Source: CAD feature listing. Evaluate the final solid. Frame: model axes, mm. A direction names the side the tool comes from. Give positions to 0.01 mm unless a question says otherwise; leave off trailing zeros. Loops run counter-clockwise (first coordinate to the right, second up) from the corner with the lowest first, then second, coordinate; pieces in that order, holes last. Notation, with made-up numbers: (40, -21) -> (83, -21) arc R9 cw to (83, -4) -> close; hole circle Ø10 at (44, -22). An arc over 180 degrees is marked (long way). Return JSON: item names as keys, results as strings. Group by question number.
```python
from build123d import *

# Parameters (mm, degrees)
SKETCH_1_W          = 25
SKETCH_1_H          = 10
EXTRUDE_1_DEPTH     = 3
EXTRUDE_3_DEPTH     = 7
EXTRUDE_4_DEPTH     = 39
EXTRUDE_6_DEPTH     = 3
EXTRUDE_7_DEPTH     = 3
SKETCH_10_W         = 25
SKETCH_10_H         = 10
CUT_EXTRUDE_1_DEPTH = 3
FILLET_1_R          = 5
FILLET_2_R          = 5
SKETCH_12_W         = 9
SKETCH_12_H         = 1.5
EXTRUDE_9_DEPTH     = 4
FILLET_3_R          = 5


with BuildPart() as part:
    # 草图1 → 凸台-拉伸1 (new body)
    with BuildSketch(Plane.XY):
        with Locations((12.5, -5)):
            Rectangle(SKETCH_1_W, SKETCH_1_H)
    extrude(amount=EXTRUDE_1_DEPTH)

    # 草图5 → 凸台-拉伸3 (add)
    with BuildSketch(Plane.XY.offset(3)):
        Polygon((25, 0), (-2, 0), (-8, 0), (-8, -3), (0, -3), (27.572478777, -3), (31, -3), (31, 0), align=None)
    extrude(amount=EXTRUDE_3_DEPTH)

    # 草图6 → 凸台-拉伸4 (add)
    with BuildSketch(Plane(origin=(31, 0, 0), x_dir=(0, 0, -1), z_dir=(1, 0, 0))):
        Polygon((-10, 0), (-25.384776311, 15.384776311), (-29.142135624, 15.384776311), (-29.142135624, 18.384776311), (-24.142135624, 18.384776311), (-5.757359313, 0), align=None)
    extrude(amount=-EXTRUDE_4_DEPTH)

    # 草图8 → 凸台-拉伸6 (add)
    with BuildSketch(Plane(origin=(31, 0, 0), x_dir=(0, 0, -1), z_dir=(1, 0, 0))):
        Polygon((-29.142135624, 15.384776311), (-25.384776311, 15.384776311), (-10, 0), (-10, -3), (-29.142135624, -3), align=None)
    extrude(amount=-EXTRUDE_6_DEPTH)

    # 草图9 → 凸台-拉伸7 (add)
    with BuildSketch(Plane.ZY.offset(8)):
        Polygon((29.142135624, 15.384776311), (25.384776311, 15.384776311), (10, 0), (10, -3), (29.142135624, -3), align=None)
    extrude(amount=-EXTRUDE_7_DEPTH)

    # 草图10 → 切除-拉伸1 (cut)
    with BuildSketch(Plane(origin=(0, 0, 0), x_dir=(-1, 0, 0), z_dir=(0, 0, -1))):
        with Locations((-12.5, -5)):
            Rectangle(SKETCH_10_W, SKETCH_10_H)
    extrude(amount=-CUT_EXTRUDE_1_DEPTH, mode=Mode.SUBTRACT)

    # 圆角1
    fillet_1_edges = [part.edges().sort_by_distance(p)[0] for p in [
        (11.5, 18.384776311, 24.142135624),
    ]]
    fillet(fillet_1_edges, radius=FILLET_1_R)

    # 圆角2
    fillet_2_edges = [part.edges().sort_by_distance(p)[0] for p in [
        (11.5, 0, 5.757359313),
    ]]
    fillet(fillet_2_edges, radius=FILLET_2_R)

    # 草图12 → 凸台-拉伸9 (add)
    with BuildSketch(Plane(origin=(0, 15.384776311, 0), x_dir=(-1, 0, 0), z_dir=(0, -1, 0))):
        with Locations((-11.5, -28.392135624)):
            Rectangle(SKETCH_12_W, SKETCH_12_H)
    extrude(amount=EXTRUDE_9_DEPTH)

    # 圆角3
    # the kernel refuses this fillet: 5 mm, written as the material it takes off along each edge
    with BuildSketch(Plane(origin=(16, 11.384776311, 41.389584338), x_dir=(-1.590727549682408e-12, 1.0, 0), z_dir=(0, 0, -1))) as fillet_3_piece_1_section:
        with BuildLine():
            CenterArc((5, -4.898979486), FILLET_3_R, 101.536959033, 78.463040967)
            Line((0, -4.898979486), (0, 0))
            Line((0, 0), (4, 0))
        make_face()
    fillet_3_piece_1 = extrude(amount=25.994897428, mode=Mode.PRIVATE)
    fillet_3_piece_1 = split(fillet_3_piece_1, bisect_by=Plane(origin=(14.26962273, 15.448091311, 25.448091311), z_dir=(0, -0.7071067811865475, 0.7071067811865476)), keep=Keep.TOP, mode=Mode.PRIVATE)
    add(fillet_3_piece_1, mode=Mode.SUBTRACT)
    with BuildSketch(Plane(origin=(7, 11.384776311, 15.39468691), x_dir=(1.5905055050774829e-12, 1.0, 0), z_dir=(0, 0, 1))) as fillet_3_piece_2_section:
        with BuildLine():
            CenterArc((5, -4.898979486), FILLET_3_R, 101.536959033, 78.463040967)
            Line((0, -4.898979486), (0, 0))
            Line((0, 0), (4, 0))
        make_face()
    fillet_3_piece_2 = extrude(amount=25.994897428, mode=Mode.PRIVATE)
    fillet_3_piece_2 = split(fillet_3_piece_2, bisect_by=Plane(origin=(8.73037727, 15.448091311, 25.448091311), z_dir=(0, -0.7071067811865475, 0.7071067811865476)), keep=Keep.TOP, mode=Mode.PRIVATE)
    add(fillet_3_piece_2, mode=Mode.SUBTRACT)


solid = part.part
```
1) Cut plane C-C on z = 20.5. Return loops of the section in (x, y), then the cut area to 3 significant figures.
2) Contact query for flat-ended pins moving along their axis: P1, Ø3, axis at x = 14.5, z = 27, coming from the -Y side; P2, Ø1, axis at x = 6.5, z = 18, coming from the -Y side; P3, Ø10, axis at x = 13.5, z = 11.5, coming from the +Y side. Output: stop coordinate, or through.
3) Mould query, pull axis X, two halves, no side actions, for faces 1 (the face through (-8, 5, 19)), 2 (the face through (11, -1, 10)), 3 (the face through (10, 12, 29.142)). Classes: released by +X, released by -X, zero draft, split by the parting line, or undercut.
4) Material intervals for line 1 (X direction, y = 3.25, z = 17.75); line 2 (Y direction, x = 21, z = 8.75); line 3 (Y direction, x = 4.5, z = 26), sorted ascending.
5) Reachability of faces 4 (the face through (11.23, 17.99, 24.27)), 5 (the face through (12, 15.385, 27)), 6 (the face through (28, 4, 22)) from +Z, -Z, +X, -X, +Y, -Y: full face, straight path, thin tool, end or side. Return the list, or none.
6) Cut plane A-A on y = -1.5. Return loops of the section in (x, z).
7) Cut plane D-D on z = 5. Return loops of the section in (x, y).
8) Cut plane B-B on x = 27.5. Return loops of the section in (y, z), then the cut area to 3 significant figures.
Calculated:
{
 "1": {"outline": "(-8, -3) -> (-5, -3) -> (-5, 10.5) -> (28, 10.5) -> (28, -3) -> (31, -3) -> (31, 14.74) -> (-8, 14.74) -> close", "area": "246 mm2"},
 "2": {"P1": "y = 11.82", "P2": "y = 7.5", "P3": "y = 10.74"},
 "3": {"face 1": "released by -X", "face 2": "undercut", "face 3": "zero draft"},
 "4": {"line 1": "-8 to -5, 28 to 31", "line 2": "-3 to 2.99", "line 3": "15.38 to 18.38"},
 "5": {"face 4": "-Z, +X, -X, +Y", "face 5": "-Y", "face 6": "+Z, -Y"},
 "6": {"outline": "(-8, 3) -> (31, 3) -> (31, 29.14) -> (28, 29.14) -> (28, 10) -> (-5, 10) -> (-5, 29.14) -> (-8, 29.14) -> close"},
 "7": {"outline": "(-8, -3) -> (31, -3) -> (31, 0.18) -> (-8, 0.18) -> close"},
 "8": {"outline": "(-3, 3) -> (0, 3) -> (0, 3.69) arc R5 cw to (1.46, 7.22) -> (16.92, 22.68) arc R5 ccw to (18.38, 26.21) -> (18.38, 29.14) -> (15.38, 29.14) -> (15.38, 25.38) -> (0, 10) -> (-3, 10) -> close", "area": "106 mm2"}
}
